Read the model definition and answer for the solid it produces. Units are mm, in the model's axes. Face numbers are marked on the shaded views. A direction names the side the tool comes from. Coordinates: 2 decimals unless noted, no trailing zeros. Write each loop counter-clockwise with the first axis right and the second up, starting at its lowest first coordinate (ties: lowest second). Pieces come first, ordered by that corner, then holes. Notation, with made-up numbers: (79.25, -39) -> (100.25, -39) arc R7 cw to (100.25, -29) -> close; hole circle Ø4 at (62.5, -35.5). An arc over 180 degrees is marked (long way). Write item = value, one per line. Start each with the question number.
1) Section A-A (z = 11.5) is taken. Count the separate pieces of the cut face and the enclosed holes in it, plus the area to 3 significant figures.
2) For a pull along Y with two mould halves and no side action, classify the marked faces 6, 7 and 8 as released by +Y, released by -Y, zero draft, split by the parting line, or undercut.
3) Flat-ended cylindrical pins translate along their axes: pin 1 Ø0.8 at (y, z) = (-33, -6.5) entering from -X; pin 2 Ø2.5 at (y, z) = (-9, 4.5) entering from -X; pin 3 Ø1 at (y, z) = (-22.5, -4.5) entering from +X; pin 4 Ø1 at (y, z) = (-41.5, 14) entering from +X. Find the tip coordinate at first contact, or state that the pin passes through.
4) A tool of negligible diameter and unlimited length cuts with its end or side. For the marked faces 1, 2, 3, 4 and 5, from which of +Z, -Z, +X, -X, +Y, -Y can it reach the whole face along a straight path? Write none if from no direction.
5) Find the intervals of material crossed by line 1 along Y through (x, z) = (10.5, 4); line 2 along Z through (x, y) = (-4.5, -27); line 3 along X through (y, z) = (-24.5, 17), in increasing order. Write a range as from..to.
6) Section D-D (x = 18.5) is taken. Determine the outline of the cut face in (y, z).
7) Section C-C (y = -27.5) is taken. Determine the outline of the cut face in (x, z).
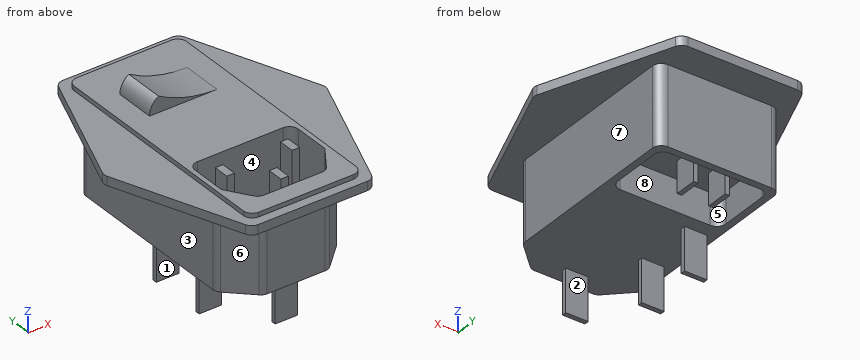
from build123d import *

# Parameters (mm, degrees)
EXTRUDE_1_DEPTH     = 17.5
EXTRUDE_2_DEPTH     = 2
SKETCH_3_W          = 25
SKETCH_3_H          = 55.25
EXTRUDE_3_DEPTH     = 1
FILLET_1_R          = 2
FILLET_2_R          = 2
FILLET_3_R          = 2
SKETCH_4_W          = 15
SKETCH_4_H          = 9
EXTRUDE_4_DEPTH     = 3.5
CUT_EXTRUDE_1_DEPTH = 9
SKETCH_6_W          = 1.7
SKETCH_6_H          = 3.5
CUT_EXTRUDE_2_DEPTH = 18
FILLET_4_R          = 2
CUT_EXTRUDE_3_DEPTH = 7
SKETCH_8_W          = 5
SKETCH_8_H          = 1
EXTRUDE_5_DEPTH     = 9.5
SKETCH_9_W          = 1
SKETCH_9_H          = 5
EXTRUDE_6_DEPTH     = 7


with BuildPart() as part:
    # Эскиз1 → Бобышка-Вытянуть1 (new body)
    with BuildSketch(Plane.XY):
        Polygon((0, 0), (27, 0), (27, -41.25), (20.75, -47.25), (6.25, -47.25), (0, -41.25), align=None)
    extrude(amount=EXTRUDE_1_DEPTH)

    # Эскиз2 → Бобышка-Вытянуть2 (add)
    with BuildSketch(Plane.XY.offset(17.5)):
        Polygon((0, 7), (27, 7), (38.25, -22.625), (27, -52.25), (0, -52.25), (-11.25, -22.625), align=None)
    extrude(amount=EXTRUDE_2_DEPTH)

    # Эскиз3 → Бобышка-Вытянуть3 (add)
    with BuildSketch(Plane.XY.offset(19.5)):
        with Locations((13.5, -22.625)):
            Rectangle(SKETCH_3_W, SKETCH_3_H)
    extrude(amount=EXTRUDE_3_DEPTH)

    # Скругление1
    fillet_1_edges = [part.edges().sort_by_distance(p)[0] for p in [
        (0, 7, 18.5),
        (27, -52.25, 18.5),
        (38.25, -22.625, 18.5),
        (27, 7, 18.5),
    ]]
    fillet(fillet_1_edges, radius=FILLET_1_R)

    # Скругление2
    fillet_2_edges = [part.edges().sort_by_distance(p)[0] for p in [
        (-11.25, -22.625, 18.5),
        (0, -52.25, 18.5),
    ]]
    fillet(fillet_2_edges, radius=FILLET_2_R)

    # Скругление3
    fillet_3_edges = [part.edges().sort_by_distance(p)[0] for p in [
        (1, 5, 20),
        (1, -50.25, 20),
        (26, -50.25, 20),
        (26, 5, 20),
    ]]
    fillet(fillet_3_edges, radius=FILLET_3_R)

    # Эскиз4 → Бобышка-Вытянуть4 (add)
    with BuildSketch(Plane.XY.offset(20.5)):
        with Locations((13.5, -8.5)):
            Rectangle(SKETCH_4_W, SKETCH_4_H)
    extrude(amount=EXTRUDE_4_DEPTH)

    # Эскиз5 → Вырез-Вытянуть1 (cut)
    with BuildSketch(Plane(origin=(0, -4, 0), x_dir=(1, 0, 0), z_dir=(0, 1, 0))):
        with BuildLine():
            ThreePointArc((21, -20.5), (14.268543991, -21.390306253), (8, -24))
            Line((8, -24), (21, -24))
            Line((21, -24), (21, -20.5))
        make_face()
        with BuildLine():
            Line((6, -20.5), (6, -24))
            Line((6, -24), (8, -24))
            ThreePointArc((8, -24), (6.535262235, -22.515564437), (6, -20.5))
        make_face()
    extrude(amount=-CUT_EXTRUDE_1_DEPTH, mode=Mode.SUBTRACT)

    # Эскиз6 → Вырез-Вытянуть2 (cut)
    with BuildSketch(Plane.XY.offset(20.5)):
        with BuildLine():
            Line((4, -30.25), (23, -30.25))
            ThreePointArc((23, -30.25), (24.414213562, -30.835786438), (25, -32.25))
            Line((25, -32.25), (25, -40.25))
            Line((25, -40.25), (21.593733072, -45.359400392))
            ThreePointArc((21.593733072, -45.359400392), (20.873348334, -46.013349198), (19.929632483, -46.25))
            Line((19.929632483, -46.25), (7.070367517, -46.25))
            ThreePointArc((7.070367517, -46.25), (6.126651666, -46.013349198), (5.406266928, -45.359400392))
            Line((5.406266928, -45.359400392), (2, -40.25))
            Line((2, -40.25), (2, -32.25))
            ThreePointArc((2, -32.25), (2.585786438, -30.835786438), (4, -30.25))
        make_face()
        with Locations((6.256266928, -35.5)):
            Rectangle(SKETCH_6_W, SKETCH_6_H, mode=Mode.SUBTRACT)
        with Locations((20.743733072, -35.5)):
            Rectangle(SKETCH_6_W, SKETCH_6_H, mode=Mode.SUBTRACT)
        with Locations((13.5, -42)):
            Rectangle(SKETCH_6_W, SKETCH_6_H, mode=Mode.SUBTRACT)
    extrude(amount=-CUT_EXTRUDE_2_DEPTH, mode=Mode.SUBTRACT)

    # Скругление4
    fillet_4_edges = [part.edges().sort_by_distance(p)[0] for p in [
        (0, 0, 8.75),
        (27, 0, 8.75),
        (27, -41.25, 8.75),
        (20.75, -47.25, 8.75),
        (6.25, -47.25, 8.75),
        (0, -41.25, 8.75),
    ]]
    fillet(fillet_4_edges, radius=FILLET_4_R)

    # Эскиз7 → Вырез-Вытянуть3 (cut)
    with BuildSketch(Plane(origin=(0, 0, 0), x_dir=(-1, 0, 0), z_dir=(0, 0, -1))):
        with BuildLine():
            Line((-23.5, -1.5), (-3.5, -1.5))
            ThreePointArc((-3.5, -1.5), (-2.085786438, -2.085786438), (-1.5, -3.5))
            Line((-1.5, -3.5), (-1.5, -14.5))
            ThreePointArc((-1.5, -14.5), (-2.085786438, -15.914213562), (-3.5, -16.5))
            Line((-3.5, -16.5), (-23.5, -16.5))
            ThreePointArc((-23.5, -16.5), (-24.914213562, -15.914213562), (-25.5, -14.5))
            Line((-25.5, -14.5), (-25.5, -3.5))
            ThreePointArc((-25.5, -3.5), (-24.914213562, -2.085786438), (-23.5, -1.5))
        make_face()
    extrude(amount=-CUT_EXTRUDE_3_DEPTH, mode=Mode.SUBTRACT)

    # Эскиз8 → Бобышка-Вытянуть5 (add)
    with BuildSketch(Plane(origin=(0, 0, 0), x_dir=(-1, 0, 0), z_dir=(0, 0, -1))):
        with Locations((-4.5, -20)):
            Rectangle(SKETCH_8_W, SKETCH_8_H)
        with Locations((-4.5, -33)):
            Rectangle(SKETCH_8_W, SKETCH_8_H)
        with Locations((-13.5, -43.75)):
            Rectangle(SKETCH_8_W, SKETCH_8_H)
    extrude(amount=EXTRUDE_5_DEPTH)

    # Эскиз9 → Бобышка-Вытянуть6 (add)
    with BuildSketch(Plane(origin=(0, 0, 7), x_dir=(-1, 0, 0), z_dir=(0, 0, -1))):
        with Locations((-7, -9)):
            Rectangle(SKETCH_9_W, SKETCH_9_H)
        with Locations((-14, -9)):
            Rectangle(SKETCH_9_W, SKETCH_9_H)
    extrude(amount=EXTRUDE_6_DEPTH)


solid = part.part
Answer key:
q1.separate_pieces = 4
q1.enclosed_holes = 1
q1.area = 912 mm^2
q2.face_6 = released by -Y
q2.face_7 = zero draft
q2.face_8 = undercut
q3.pin_1 = 2
q3.pin_2 = 0
q3.pin_3 = through
q3.pin_4 = 26.91
q4.face_1 = -Z, +X, -X
q4.face_2 = -Z, +X, -X, +Y
q4.face_3 = -Z, -X, +Y, -Y
q4.face_4 = +Z
q4.face_5 = -Z
q5.line_1 = -47.25..-46.25, -30.25..-16.5, -1.5..0
q5.line_2 = 17.5..19.5
q5.line_3 = 0..27
q6.outline = (-52.25, 17.5) -> (-47.25, 17.5) -> (-47.25, 0) -> (-16.5, 0) -> (-16.5, 7) -> (-1.5, 7) -> (-1.5, 0) -> (0, 0) -> (0, 17.5) -> (7, 17.5) -> (7, 19.5) -> (5, 19.5) -> (5, 20.5) -> (-4, 20.5) -> (-4, 20.62) -> (-13, 20.62) -> (-13, 20.5) -> (-30.25, 20.5) -> (-30.25, 2.5) -> (-46.25, 2.5) -> (-46.25, 20.5) -> (-50.25, 20.5) -> (-50.25, 19.5) -> (-52.25, 19.5) -> close
q7.outline = (-9.4, 17.5) -> (0, 17.5) -> (0, 0) -> (27, 0) -> (27, 17.5) -> (36.4, 17.5) -> (36.4, 19.5) -> (26, 19.5) -> (26, 20.5) -> (1, 20.5) -> (1, 19.5) -> (-9.4, 19.5) -> close
